```python
from build123d import *
from OCP.BRepFilletAPI import BRepFilletAPI_MakeChamfer

# Parameters (mm, degrees)
SKETCH1_W           = 28
SKETCH1_H           = 27
BOSS_EXTRUDE1_DEPTH = 2
SKETCH2_W           = 10
SKETCH2_H           = 2.5
CUT_EXTRUDE1_DEPTH  = 2
SKETCH3_W           = 20
SKETCH3_H           = 14.5
BOSS_EXTRUDE2_DEPTH = 3
SKETCH4_W           = 24
SKETCH4_H           = 23
SKETCH4_W_2         = 20
SKETCH4_H_2         = 19
BOSS_EXTRUDE3_DEPTH = 6
SKETCH5_R           = 0.95
CUT_EXTRUDE2_DEPTH  = 3.2
FILLET1_R           = 2
FILLET2_R           = 0.5
CHAMFER1_SIZE       = 3.5
CHAMFER1_SIZE2      = 0.306210322


with BuildPart() as part:
    # Sketch1 → Boss-Extrude1 (new body)
    with BuildSketch(Plane(origin=(0, 0, 0), x_dir=(1, 0, 0), z_dir=(0, 1, 0))):
        Rectangle(SKETCH1_W, SKETCH1_H)
    extrude(amount=BOSS_EXTRUDE1_DEPTH)

    # Sketch2 → Cut-Extrude1 (cut)
    with BuildSketch(Plane(origin=(0, 2, 0), x_dir=(1, 0, 0), z_dir=(0, 1, 0))):
        with Locations((3, 7.25)):
            Rectangle(SKETCH2_W, SKETCH2_H)
    extrude(amount=-CUT_EXTRUDE1_DEPTH, mode=Mode.SUBTRACT)

    # Sketch3 → Boss-Extrude2 (add)
    with BuildSketch(Plane(origin=(0, 2, 0), x_dir=(1, 0, 0), z_dir=(0, 1, 0))):
        with Locations((0, -2.25)):
            Rectangle(SKETCH3_W, SKETCH3_H)
    extrude(amount=BOSS_EXTRUDE2_DEPTH)

    # Sketch4 → Boss-Extrude3 (add)
    with BuildSketch(Plane(origin=(0, 2, 0), x_dir=(1, 0, 0), z_dir=(0, 1, 0))):
        Rectangle(SKETCH4_W, SKETCH4_H)
        Rectangle(SKETCH4_W_2, SKETCH4_H_2, mode=Mode.SUBTRACT)
    extrude(amount=BOSS_EXTRUDE3_DEPTH)

    # Sketch5 → Cut-Extrude2 (cut)
    with BuildSketch(Plane(origin=(0, 5, 0), x_dir=(1, 0, 0), z_dir=(0, 1, 0))):
        with Locations(Location((-7, -6.5, 0), (0, 0, 270))):
            Circle(SKETCH5_R)
        with Locations(Location((7, -6.5, 0), (0, 0, 90))):
            Circle(SKETCH5_R)
    extrude(amount=-CUT_EXTRUDE2_DEPTH, mode=Mode.SUBTRACT)

    # Fillet1
    fillet1_edges = [part.edges().sort_by_distance(p)[0] for p in [
        (12, 5, -11.5),
        (-12, 5, -11.5),
        (-12, 5, 11.5),
        (12, 5, 11.5),
        (14, 1, 13.5),
        (-14, 1, 13.5),
        (-14, 1, -13.5),
        (14, 1, -13.5),
    ]]
    fillet(fillet1_edges, radius=FILLET1_R)

    # Fillet2
    fillet2_edges = [part.edges().sort_by_distance(p)[0] for p in [
        (-2, 1, -8.5),
        (-2, 1, -6),
        (8, 1, -6),
        (8, 1, -8.5),
        (10, 5, -9.5),
        (-10, 6.5, 9.5),
        (10, 6.5, 9.5),
        (-10, 5, -9.5),
    ]]
    fillet(fillet2_edges, radius=FILLET2_R)

    # Chamfer1: one chamfer whose edges measure the first distance from different faces: ONE call of the kernel's chamfer builder (chamfer() names one face for all edges)
    chamfer1_edges_1 = [part.edges().sort_by_distance(p)[0] for p in [
        (0, 8, -11.5),
    ]]
    chamfer1_side_1 = [part.faces().sort_by_distance(p)[0] for p in [
        (0, 5, -11.5),
    ]]
    chamfer1_edges_2 = [part.edges().sort_by_distance(p)[0] for p in [
        (12, 8, 0),
    ]]
    chamfer1_side_2 = [part.faces().sort_by_distance(p)[0] for p in [
        (12, 5, 0),
    ]]
    chamfer1_edges_3 = [part.edges().sort_by_distance(p)[0] for p in [
        (-12, 8, 0),
    ]]
    chamfer1_side_3 = [part.faces().sort_by_distance(p)[0] for p in [
        (-12, 5, 0),
    ]]
    chamfer1_edges_4 = [part.edges().sort_by_distance(p)[0] for p in [
        (0, 8, 11.5),
    ]]
    chamfer1_side_4 = [part.faces().sort_by_distance(p)[0] for p in [
        (0, 5, 11.5),
    ]]
    chamfer1_edges_5 = [part.edges().sort_by_distance(p)[0] for p in [
        (-11.414213562, 8, -10.914213562),
    ]]
    chamfer1_side_5 = [part.faces().sort_by_distance(p)[0] for p in [
        (-11.414213562, 5, -10.914213562),
    ]]
    chamfer1_edges_6 = [part.edges().sort_by_distance(p)[0] for p in [
        (-11.414213562, 8, 10.914213562),
    ]]
    chamfer1_side_6 = [part.faces().sort_by_distance(p)[0] for p in [
        (-11.414213562, 5, 10.914213562),
    ]]
    chamfer1_edges_7 = [part.edges().sort_by_distance(p)[0] for p in [
        (11.414213562, 8, 10.914213562),
    ]]
    chamfer1_side_7 = [part.faces().sort_by_distance(p)[0] for p in [
        (11.414213562, 5, 10.914213562),
    ]]
    chamfer1_edges_8 = [part.edges().sort_by_distance(p)[0] for p in [
        (11.414213562, 8, -10.914213562),
    ]]
    chamfer1_side_8 = [part.faces().sort_by_distance(p)[0] for p in [
        (11.414213562, 5, -10.914213562),
    ]]
    chamfer1 = BRepFilletAPI_MakeChamfer(part.part.solid().wrapped)
    for e in chamfer1_edges_1:
        chamfer1.Add(CHAMFER1_SIZE, CHAMFER1_SIZE2, e.wrapped, chamfer1_side_1[0].wrapped)  # the first distance lies on this face
    for e in chamfer1_edges_2:
        chamfer1.Add(CHAMFER1_SIZE, CHAMFER1_SIZE2, e.wrapped, chamfer1_side_2[0].wrapped)  # the first distance lies on this face
    for e in chamfer1_edges_3:
        chamfer1.Add(CHAMFER1_SIZE, CHAMFER1_SIZE2, e.wrapped, chamfer1_side_3[0].wrapped)  # the first distance lies on this face
    for e in chamfer1_edges_4:
        chamfer1.Add(CHAMFER1_SIZE, CHAMFER1_SIZE2, e.wrapped, chamfer1_side_4[0].wrapped)  # the first distance lies on this face
    for e in chamfer1_edges_5:
        chamfer1.Add(CHAMFER1_SIZE, CHAMFER1_SIZE2, e.wrapped, chamfer1_side_5[0].wrapped)  # the first distance lies on this face
    for e in chamfer1_edges_6:
        chamfer1.Add(CHAMFER1_SIZE, CHAMFER1_SIZE2, e.wrapped, chamfer1_side_6[0].wrapped)  # the first distance lies on this face
    for e in chamfer1_edges_7:
        chamfer1.Add(CHAMFER1_SIZE, CHAMFER1_SIZE2, e.wrapped, chamfer1_side_7[0].wrapped)  # the first distance lies on this face
    for e in chamfer1_edges_8:
        chamfer1.Add(CHAMFER1_SIZE, CHAMFER1_SIZE2, e.wrapped, chamfer1_side_8[0].wrapped)  # the first distance lies on this face
    add(Compound.cast(chamfer1.Shape()), mode=Mode.REPLACE)


solid = part.part
```
Verification items for the finished model (mm, model axes). A direction names the side the tool comes from. Give positions to 0.01 mm unless a question says otherwise; leave off trailing zeros. Order: outer loops, then holes, each group sorted by start corner. A loop starts at its lowest first (then second) coordinate and runs counter-clockwise, first axis right, second up. Notation, with made-up numbers: (17, 22.25) -> (24, 22.25) arc R13 cw to (24, 39.25) -> close; hole circle Ø8 at (5.25, -22.75). An arc over 180 degrees is marked (long way). One line per item, written item: value.
(1) Sectioned sample at D-D on x = -7. Record the cut outline in (y, z), then the cut area to 3 significant figures.
Final values:
outline: (0, -13.5) -> (2, -13.5) -> (2, -11.5) -> (4.5, -11.5) -> (8, -11.19) -> (8, -9.5) -> (2, -9.5) -> (2, -5) -> (5, -5) -> (5, 5.55) -> (1.8, 5.55) -> (1.8, 7.45) -> (5, 7.45) -> (5, 9.5) -> (8, 9.5) -> (8, 11.19) -> (4.5, 11.5) -> (2, 11.5) -> (2, 13.5) -> (0, 13.5) -> close
area: 114 mm^2
(2) Sectioned sample at B-B on z = 8.25. Record the cut outline in (x, y).
Final values:
outline: (-14, 0) -> (14, 0) -> (14, 2) -> (12, 2) -> (12, 4.5) -> (11.69, 8) -> (10, 8) -> (10, 5) -> (-10, 5) -> (-10, 8) -> (-11.69, 8) -> (-12, 4.5) -> (-12, 2) -> (-14, 2) -> close
(3) Scan lines: line 1 along Z through (x, y) = (7, 2.85); line 2 along X through (y, z) = (3.3, 6.5); line 3 along Y through (x, z) = (12.25, -11). Record each from-to range of solid material in increasing order. Write a range as [from, to].
Final values:
line 1: [-11.5, -9.5], [-5, 5.55], [7.45, 11.5]
line 2: [-12, -7.95], [-6.05, 6.05], [7.95, 12]
line 3: [0, 2]
(4) Tool access check on faces 1 (the face through (11.4, 3.27, -10.93)), 2 (the face through (12, 3, 0)), 3 (the face through (7, 1.8, 7)). Record the directions out of +Z, -Z, +X, -X, +Y, -Y that give a thin tool (end or side, any length) a straight path to the whole face; none if there is none.
Final values:
face 1: -Z, +X, +Y
face 2: +Z, -Z, +X, +Y
face 3: +Y
(5) Sectioned sample at C-C on y = 5.5. Record the cut outline in (x, z).
Final values:
outline: (-11.91, -9.5) arc R1.91 ccw to (-10, -11.41) -> (10, -11.41) arc R1.91 ccw to (11.91, -9.5) -> (11.91, 9.5) arc R1.91 ccw to (10, 11.41) -> (-10, 11.41) arc R1.91 ccw to (-11.91, 9.5) -> close; hole (-10, -9) arc R0.5 ccw to (-9.5, -9.5) -> (9.5, -9.5) arc R0.5 ccw to (10, -9) -> (10, 9) arc R0.5 ccw to (9.5, 9.5) -> (-9.5, 9.5) arc R0.5 ccw to (-10, 9) -> close
(6) Gauge pin test, flat ends, axial feed: pin 1 (4 mm diameter, centred on x = -9.5, y = 6.5, fed in from +Z); pin 2 (1.5 mm diameter, centred on y = 3, z = 8.5, fed in from -X); pin 3 (1.5 mm diameter, centred on x = -6.5, z = 7, fed in from +Y). Record the tip position at first contact, or that the pin passes through.
Final values:
pin 1: z = 11.5
pin 2: x = -12
pin 3: y = 5
(7) Sectioned sample at A-A on x = 7. Record the cut outline in (y, z).
Final values:
outline: (0, -13.5) -> (2, -13.5) -> (2, -11.5) -> (4.5, -11.5) -> (8, -11.19) -> (8, -9.5) -> (2, -9.5) -> (2, -8.5) -> (0, -8.5) -> close; (0, -6) -> (2, -6) -> (2, -5) -> (5, -5) -> (5, 5.55) -> (1.8, 5.55) -> (1.8, 7.45) -> (5, 7.45) -> (5, 9.5) -> (8, 9.5) -> (8, 11.19) -> (4.5, 11.5) -> (2, 11.5) -> (2, 13.5) -> (0, 13.5) -> close
(8) Draft check along Z on faces 4 (the face through (-11.43, 3.27, 10.9)), 5 (the face through (3, 1, -8.5)), 6 (the face through (11.845, 6.274, -0.133)). Enter one of: pulls with the +Z half, pulls with the -Z half, needs draft (parallel to the pull), parting line crosses it, or undercut.
Final values:
face 4: pulls with the +Z half
face 5: undercut
face 6: needs draft
